Source: CAD feature listing. Evaluate the final solid. Frame: model axes, mm. A direction names the side the tool comes from. Coordinates: 2 decimals unless noted, no trailing zeros. Order: outer loops, then holes, each group sorted by start corner. A loop starts at its lowest first (then second) coordinate and runs counter-clockwise, first axis right, second up.
```python
from build123d import *

# Parameters (mm, degrees)
SKETCH_1_R          = 15
EXTRUDE_1_DEPTH     = 205.5
SKETCH_2_R          = 15
SKETCH_2_R_2        = 12.5
CUT_EXTRUDE_1_DEPTH = 86


# Read off the part's stored shape, not the designer's step: 切除-旋转3
with BuildPart() as part:
    # 草图1 → 凸台-拉伸1 (new, symmetric)
    with BuildSketch(Plane.XY):
        Circle(SKETCH_1_R)
    extrude(amount=EXTRUDE_1_DEPTH, both=True)

    # 草图2 → 切除-拉伸1 (cut)
    with BuildSketch(Plane.XY.offset(205.5)):
        Circle(SKETCH_2_R)
        Circle(SKETCH_2_R_2, mode=Mode.SUBTRACT)
    extrude(amount=-CUT_EXTRUDE_1_DEPTH, mode=Mode.SUBTRACT)

    # 切除-旋转3 outline → 切除-旋转3 (revolve, cut)
    with BuildSketch(Plane.XZ):
        Polygon((15, -155.5), (12.5, -205.5), (15, -205.5), align=None)
    revolve(axis=Axis((0, 0, 0), (0, 0, 1)), mode=Mode.SUBTRACT)


solid = part.part
```
1. Section query A-A, the plane x = 0. Output: boundary loops of the cut face in (y, z).
2. Contact query for flat-ended pins moving along their axis: P1, Ø5, axis at x = 8.5, z = 0.5, coming from the -Y side; P2, Ø2, axis at x = 5.5, z = 90, coming from the -Y side; P3, Ø8, axis at x = -10.5, z = 98, coming from the -Y side. Output: stop coordinate, or through.
3. Access query for faces 1 (the cylindrical face through (11.923, 3.755, 163.102)), 2 (the flat face through (0, 0, -205.5)). Directions: +Z, -Z, +X, -X, +Y, -Y. A direction counts if a zero-diameter tool reaches every point of the face in a straight line with its end or side. Return the directions, or none.
4. Material intervals for line 1 along X through (y, z) = (-0.75, 88.5); line 2 along Y through (x, z) = (-8.25, 114); line 3 along X through (y, z) = (10.75, -1), sorted ascending.
5. Section query C-C, the plane z = -50.5. Output: boundary loops of the cut face in (x, y).
6. Section query D-D, the plane z = -167.5. Output: boundary loops of the cut face in (x, y), plus the area to 3 significant figures.
Answer key:
1. outline: (-15, -155.5) - (-12.5, -205.5) - (12.5, -205.5) - (15, -155.5) - (15, 119.5) - (12.5, 119.5) - (12.5, 205.5) - (-12.5, 205.5) - (-12.5, 119.5) - (-15, 119.5) - close
2. P1: stops at y = -13.75
2. P2: stops at y = -14.31
2. P3: stops at y = -13.52
3. face 1: +Z
3. face 2: -Z, +X, -X, +Y, -Y
4. line 1: x = -14.98 to 14.98
4. line 2: y = -12.53 to 12.53
4. line 3: x = -10.46 to 10.46
5. outline: circle Ø30 at (0, 0)
6. outline: circle Ø28.8 at (0, 0)
6. area: 651 mm2
